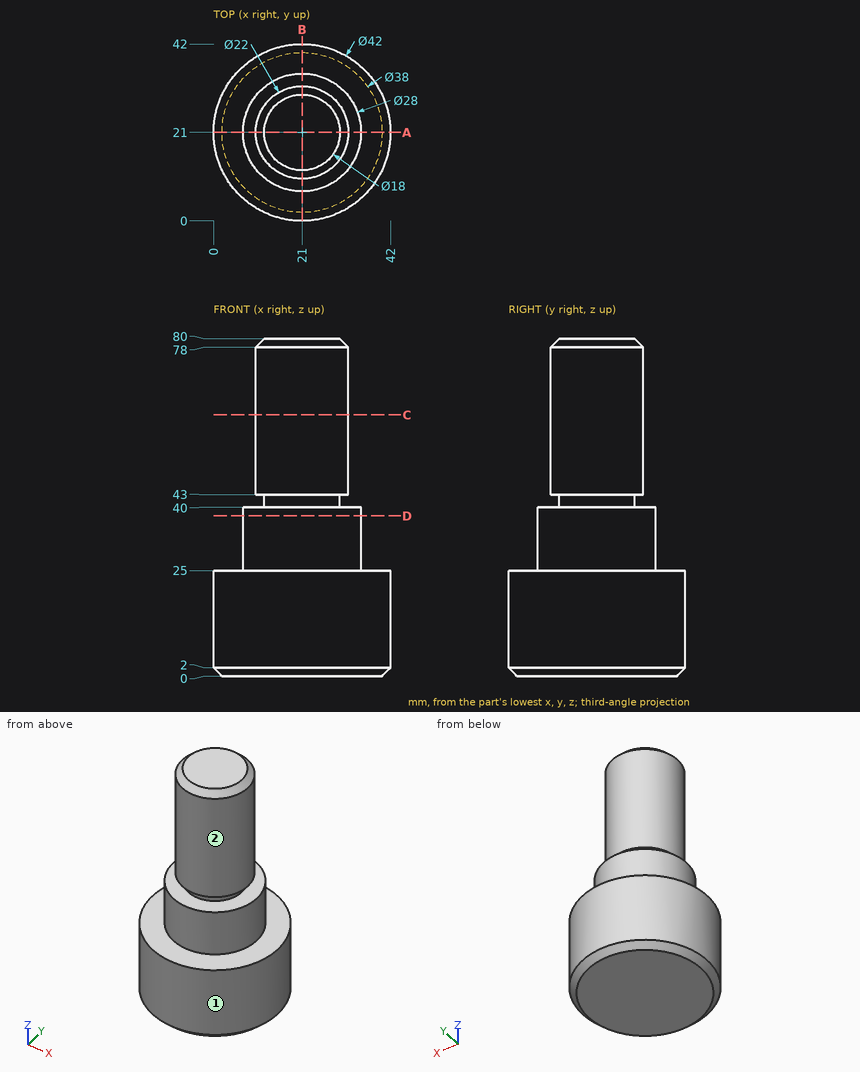
Study the drawing (mm; zero at the part's minimum x, y, z) and answer. A direction names the side the tool comes from. Round coordinates to 2 decimals unless told otherwise and drop trailing zeros. Write each loop counter-clockwise with the first axis right and the second up, starting at its lowest first coordinate (ties: lowest second). Pieces come first, ordered by that corner, then holes.
1) A cutting plane is placed at D-D on z = 38. Determine the outline of the cut face in (x, y), and give its area (3 significant figures).
2) A cutting plane is placed at C-C on z = 62. Determine the outline of the cut face in (x, y), and give its area (3 significant figures).
3) Which of the six approach directions +Z, -Z, +X, -X, +Y, -Y give full straight-line access (tool end or side, diameter ignored) to the marked faces 1 and 2?
4) A cutting plane is placed at A-A on y = 21. Determine the outline of the cut face in (x, z), and give its area (3 significant figures).
5) Consider probe 1 along Z at (x, y) = (12, 8.5); probe 2 along Y at (x, z) = (20.5, 74.5); probe 3 along X at (y, z) = (11.5, 11). Determine where each line is inside the solid, lowest interval first.
6) Flat-ended cylindrical pins translate along their axes: P1, Ø10, axis at x = 15.5, z = 62, coming from the -Y side; P2, Ø4, axis at x = 5.5, z = 24, coming from the +Y side; P3, Ø2, axis at y = 11, z = 11, coming from the +X side. Find the tip coordinate at first contact, or state that the pin passes through.
Entries:
1. outline: circle Ø28 at (21, 21)
1. area: 616 mm2
2. outline: circle Ø22 at (21, 21)
2. area: 380 mm2
3. face 1: +Z, -Z
3. face 2: +Z
4. outline: (0, 2) - (2, 0) - (40, 0) - (42, 2) - (42, 25) - (35, 25) - (35, 40) - (30, 40) - (30, 43) - (32, 43) - (32, 78) - (30, 80) - (12, 80) - (10, 78) - (10, 43) - (12, 43) - (12, 40) - (7, 40) - (7, 25) - (0, 25) - close
4. area: 2,330 mm2
5. probe 1: z = 0 to 25
5. probe 2: y = 10.01 to 31.99
5. probe 3: x = 2.27 to 39.73
6. P1: stops at y = 10.01
6. P2: stops at y = 37.09
6. P3: stops at x = 39.97
